```python
from build123d import *

# Parameters (mm, degrees)
F0_W      = 124.6
F0_H      = 61.9
F1_DEPTH  = 19.05
F2_W      = 4.953
F2_H      = 14.6315630991
F2_W_2    = 29.2449435338
F2_H_2    = 13.041177066
F2_W_3    = 29.159436468
F2_R      = 3.175
F3_DEPTH  = 13.97
F5_DEPTH  = 6.35
F6_W      = 12.7
F6_H      = 25.4
F7_DEPTH  = 12.7
F8_W      = 4.953
F8_H      = 71.0073517896
F9_DEPTH  = 3.81
F10_R     = 3.81
F11_DEPTH = 5.08
F13_DEPTH = 5.08
F14_DEPTH = 31.75
F16_W     = 13.5046280921
F16_H     = 23.5811583698
F17_DEPTH = 25.4
F18_W     = 19.2745104432
F18_H     = 5.7546193711
F19_DEPTH = 31.75
F20_W     = 14.9206416681
F20_H     = 4.7117811628
F21_DEPTH = 19.05
F22_W     = 51.0552711785
F22_H     = 10.1753515191
F22_W_2   = 51.412301138
F23_DEPTH = 12.7
F24_W     = 93.4092327952
F24_H     = 5.8380772825
F24_W_2   = 76.4692127705
F24_H_2   = 3.4473836422
F25_DEPTH = 2.54
F26_W     = 95.3170992434
F26_H     = 5.4240481682
F26_W_2   = 71.3913366199
F26_H_2   = 4.0845796466
F27_DEPTH = 2.54
F28_W     = 109.2679016292
F28_H     = 7.5388159603
F29_DEPTH = 5.08
F30_W     = 48.6481711268
F30_H     = 3.1835205168
F30_W_2   = 48.6969016492
F30_H_2   = 3.9205837529
F31_DEPTH = 5.08
F32_W     = 55.2894864231
F32_H     = 4.0775961243
F32_W_2   = 55.2933309227
F32_H_2   = 3.075633198
F33_DEPTH = 5.08


# Not quite as in the source:
# - a feature names something its author has since deleted; it is built from what else it names


with BuildPart() as f1:
    # F0 (on Top) → F1 (new body)
    with BuildSketch(Plane.XY):
        Polygon((-75.2904937168, 49.9057597088), (-75.2904937168, -50.0942402912), (-42.6597435957, -50.0942402912), (67.6151300783, -50.0942402912), (74.7095062832, -50.0942402912), (74.7095062832, 49.9057597088), (-0.2904937168, 49.9057597088), (-25.810170721, 49.9057597088), (-50.4447113996, 49.9057597088), align=None)
        with Locations((-0.2904937168, -0.0942402912)):
            Rectangle(F0_W, F0_H, mode=Mode.SUBTRACT)
    extrude(amount=F1_DEPTH)

    # F2 (on face) → F3 (cut)
    with BuildSketch(Plane.XZ.offset(50.0942402912)):
        with Locations((-60.1431414232, 10.2322226157)):
            Rectangle(F2_W, F2_H)
        with Locations((-52.6501414232, 10.2322226157)):
            Rectangle(F2_W, F2_H)
        with Locations((-20.147212787, 9.4370295992)):
            Rectangle(F2_W_2, F2_H_2)
        with Locations((20.1876896899, 9.4370295992)):
            Rectangle(F2_W_3, F2_H_2)
        with Locations((52.6363079239, 10.2322226157)):
            Rectangle(F2_W, F2_H)
        with Locations((60.1293079239, 10.2322226157)):
            Rectangle(F2_W, F2_H)
        with Locations((-44.1754937168, 12.7)):
            Circle(F2_R)
        with Locations((-0.6144937168, 6.35)):
            Circle(F2_R)
        with Locations((42.9465062832, 12.7)):
            Circle(F2_R)
        with Locations((68.3465062832, 7.8599134153)):
            Circle(F2_R)
        with Locations((-68.9404937168, 6.35)):
            Circle(F2_R)
    extrude(amount=-F3_DEPTH, mode=Mode.SUBTRACT)

    # F4 (on face) → F5 (cut)
    with BuildSketch(Plane(origin=(0, 0, 0), x_dir=(1, 0, 0), z_dir=(0, 0, -1))):
        Polygon((66.3145062832, 45.4020188174), (-67.0354937168, 45.4020188174), (-67.0354937168, 35.2429834301), (-61.1156715149, 35.2429834301), (60.9613691041, 35.2429834301), (66.3145062832, 35.2429834301), align=None)
        Polygon((-67.0354937168, 35.2429834301), (-67.0354937168, 45.4020188174), (-71.9995722175, 45.4020188174), (-71.9995722175, -45.2067597088), (-67.0354937168, -45.2067597088), (-67.0354937168, -35.52858904), align=None)
        Polygon((71.2675062832, 45.4020188174), (66.3145062832, 45.4020188174), (66.3145062832, 35.2429834301), (66.4545062832, 35.2429834301), (66.4545062832, -35.52858904), (66.4545062832, -45.2067597088), (71.2675062832, -45.2067597088), align=None)
        Polygon((60.9613691041, -35.52858904), (-67.0354937168, -35.52858904), (-67.0354937168, -45.2067597088), (66.4545062832, -45.2067597088), (66.4545062832, -35.52858904), align=None)
    extrude(amount=-F5_DEPTH, mode=Mode.SUBTRACT)

    # F6 (on face) → F7 (join)
    with BuildSketch(Plane(origin=(0, 0, 0), x_dir=(1, 0, 0), z_dir=(0, 0, -1))):
        with Locations((6.35, -62.6057597088)):
            Rectangle(F6_W, F6_H)
        with Locations((-6.35, -62.6057597088)):
            Rectangle(F6_W, F6_H)
    extrude(amount=-F7_DEPTH)

    # F8 (on face) → F9 (cut)
    with BuildSketch(Plane.XY.offset(19.05)):
        Polygon((70.0243711472, 45.754622668), (-70.5914937168, 45.754622668), (-70.5914937168, 37.4231114984), (-65.6384937168, 37.4231114984), (65.065138042, 37.4231114984), (70.0243711472, 37.4231114984), align=None)
        with Locations((-68.1149937168, 1.9194356036)):
            Rectangle(F8_W, F8_H)
        Polygon((70.0243711472, -33.5842402912), (70.0243711472, 37.4231114984), (65.065138042, 37.4231114984), (65.065138042, -33.5842402912), (69.871573916, -33.5842402912), align=None)
        Polygon((-65.6384937168, -33.5842402912), (-70.5914937168, -33.5842402912), (-70.7442909479, -33.5842402912), (-70.7442909479, -36.1242402912), (69.871573916, -36.1242402912), (69.871573916, -33.5842402912), (65.065138042, -33.5842402912), align=None)
        Polygon((69.871573916, -36.1242402912), (-70.7442909479, -36.1242402912), (0, -44.9241176248), align=None)
    extrude(amount=-F9_DEPTH, mode=Mode.SUBTRACT)

    # F10 (on face) → F11 (join)
    with BuildSketch(Plane.YZ.offset(12.7)):
        with BuildLine():
            Line((49.9057597088, 12.7), (75.3057597088, 12.7))
            ThreePointArc((75.3057597088, 12.7), (62.6057597088, 25.0247137147), (49.9057597088, 12.7))
        make_face()
        with Locations((62.6057597088, 20.32)):
            Circle(F10_R, mode=Mode.SUBTRACT)
        with Locations((62.6057597088, 20.32)):
            Circle(F10_R)
    extrude(amount=-F11_DEPTH)

    # F12 (on face) → F13 (join)
    with BuildSketch(Plane(origin=(-12.7, 0, 0), x_dir=(0, -1, 0), z_dir=(-1, 0, 0))):
        with BuildLine():
            Line((-75.3057597088, 12.7), (-49.9057597088, 12.7))
            ThreePointArc((-49.9057597088, 12.7), (-62.6057597088, 25.1906117041), (-75.3057597088, 12.7))
        make_face()
    extrude(amount=-F13_DEPTH)

    # F10 (on face) → F14 (cut)
    with BuildSketch(Plane.YZ.offset(12.7)):
        with Locations((62.6057597088, 20.32)):
            Circle(F10_R)
    extrude(amount=-F14_DEPTH, mode=Mode.SUBTRACT)

    # F16 (on face) → F17 (cut)
    with BuildSketch(Plane.XY.offset(12.7)):
        with Locations((-0.017571263, 62.7732072026)):
            Rectangle(F16_W, F16_H)
    extrude(amount=-F17_DEPTH, mode=Mode.SUBTRACT)

    # F18 (on face) → F19 (cut)
    with BuildSketch(Plane(origin=(-12.7, 0, 0), x_dir=(0, -1, 0), z_dir=(-1, 0, 0))):
        with Locations((-62.7002157271, 6.9401275832)):
            Rectangle(F18_W, F18_H)
    extrude(amount=-F19_DEPTH, mode=Mode.SUBTRACT)

    # F20 (on face) → F21 (cut)
    with BuildSketch(Plane(origin=(0, 75.3057597088, 0), x_dir=(-1, 0, 0), z_dir=(0, 1, 0))):
        with Locations((0.1047314145, 6.2031324487)):
            Rectangle(F20_W, F20_H)
    extrude(amount=-F21_DEPTH, mode=Mode.SUBTRACT)

    # F22 (on face) → F23 (cut)
    with BuildSketch(Plane(origin=(0, 49.9057597088, 0), x_dir=(-1, 0, 0), z_dir=(0, 1, 0))):
        with Locations((-43.9973082393, 9.4878289383)):
            Rectangle(F22_W, F22_H)
        with Locations((44.010556303, 9.4878289383)):
            Rectangle(F22_W_2, F22_H)
    extrude(amount=-F23_DEPTH, mode=Mode.SUBTRACT)

    # F24 (on face) → F25 (cut)
    with BuildSketch(Plane(origin=(-75.2904937168, 0, 0), x_dir=(0, -1, 0), z_dir=(-1, 0, 0))):
        with Locations((0.03618747, 6.7635682644)):
            Rectangle(F24_W, F24_H)
        with Locations((0.2549141645, 13.9791369438)):
            Rectangle(F24_W_2, F24_H_2)
    extrude(amount=-F25_DEPTH, mode=Mode.SUBTRACT)

    # F26 (on face) → F27 (cut)
    with BuildSketch(Plane.YZ.offset(74.7095062832)):
        with Locations((-1.0910946876, 6.8129759159)):
            Rectangle(F26_W, F26_H)
        with Locations((-0.289645046, 14.5612489432)):
            Rectangle(F26_W_2, F26_H_2)
    extrude(amount=-F27_DEPTH, mode=Mode.SUBTRACT)

    # F28 (on face) → F29 (cut)
    with BuildSketch(Plane.XZ.offset(-30.8557597088)):
        with Locations((-0.0406969339, 11.1216651276)):
            Rectangle(F28_W, F28_H)
    extrude(amount=-F29_DEPTH, mode=Mode.SUBTRACT)

    # F30 (on face) → F31 (cut)
    with BuildSketch(Plane.YZ.offset(-62.5904937168)):
        with Locations((-1.1887364089, 11.1167602584)):
            Rectangle(F30_W, F30_H)
        with Locations((-1.1643711478, 5.3142114775)):
            Rectangle(F30_W_2, F30_H_2)
    extrude(amount=-F31_DEPTH, mode=Mode.SUBTRACT)

    # F32 (on face) → F33 (cut)
    with BuildSketch(Plane(origin=(62.0095062832, 0, 0), x_dir=(0, -1, 0), z_dir=(-1, 0, 0))):
        with Locations((1.1272905394, 6.7439966369)):
            Rectangle(F32_W, F32_H)
        with Locations((1.1480180547, 12.1434889734)):
            Rectangle(F32_W_2, F32_H_2)
    extrude(amount=-F33_DEPTH, mode=Mode.SUBTRACT)


solid = f1.part
```
The model under review builds one solid part; all positions refer to its coordinate system, in mm. A direction names the side the tool comes from. Round coordinates to 2 decimals unless told otherwise and drop trailing zeros.
1) Tool access review of faces 1 (the face through (-72.75, 0, 14)), 2 (the face through (-67.67, -2, 11)), 3 (the face through (-62.59, -1, 9)), 4 (the face through (-7.565, 73, 6)), 5 (the face through (42.26, -43.21, 9.6)): name each direction out of +Z, -Z, +X, -X, +Y, -Y from which nothing blocks a thin tool from reaching the whole face with its end or side.
Values follow:
face 1: -X
face 2: none
face 3: +Z, -Z
face 4: +Y
face 5: -Y
2) Clearance check with flat-ended pins moving along their axes: P1, Ø1.8, axis at y = 7, z = 6.5, coming from the -X side; P2, Ø4.5, axis at x = -10.5, z = 7, coming from the -Y side; P3, Ø4, axis at x = 31, z = 4.5, coming from the +Y side. State where each tip first meets the part, or that it passes through.
Values follow:
P1: stops at x = -72.75
P2: stops at y = -36.12
P3: stops at y = 49.91
3) Consider section A-A on x = 16.5. Give the number of separate pieces and of enclosed holes in the cut face, then the cut area to 3 significant figures.
Values follow:
separate pieces: 4
enclosed holes: 0
area: 349 mm2
4) The part is to be moulded in two halves that separate along Z. For faces 6 (the face through (-6.2, -44.31, 19.05)), 7 (the face through (0, 74.564, 11)), 8 (the face through (57.653, -43, 12)), say which applies: pulls with the +Z half, pulls with the -Z half, needs draft (parallel to the pull), parting line crosses it, or undercut.
Values follow:
face 6: pulls with the +Z half
face 7: needs draft
face 8: undercut
5) Wall thickness on line 1 along Y through (x, z) = (37.5, 6); line 2 along Y through (x, z) = (42.5, 2); line 3 along X through (y, z) = (-25.5, 18): over which ranges is each line inside the solid? List them lowest first.
Values follow:
line 1: y = -50.09 to -45.4, -35.24 to -31.04, 30.86 to 35.53
line 2: y = -50.09 to -45.4, -35.24 to -31.04, 30.86 to 35.53, 45.21 to 49.91
line 3: x = -75.29 to -70.59, -65.64 to -62.59, 62.01 to 65.07, 70.02 to 74.71
